Work out the finished part from the listing and answer in its coordinate system (mm). Round coordinates to 2 decimals unless told otherwise and drop trailing zeros. Loops run counter-clockwise (first coordinate to the right, second up) from the corner with the lowest first, then second, coordinate; pieces in that order, holes last. Notation, with made-up numbers: (58, -25.75) - (80, -25.75) arc R16 cw to (80, -19.75) - close; hole circle Ø10 at (74, 70). An arc over 180 degrees is marked (long way). Answer as CSV lines item,"result". Start each with the question number.
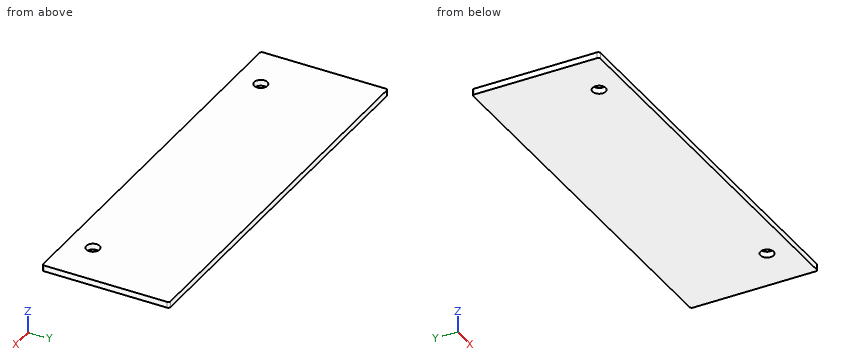
```python
from build123d import *

# Parameters (mm, degrees)
SKETCH_R  = 3.302
PAD_DEPTH = 3


with BuildPart() as part:
    # Sketch → Pad (new body)
    with BuildSketch(Plane.XY):
        with BuildLine():
            ThreePointArc((-98.21875, 31.75), (-98.925857, 31.457107), (-99.21875, 30.75))
            Line((-99.21875, -30.75), (-99.21875, 30.75))
            ThreePointArc((-99.21875, -30.75), (-98.925857, -31.457107), (-98.21875, -31.75))
            Line((98.21875, -31.75), (-98.21875, -31.75))
            ThreePointArc((98.21875, -31.75), (98.925857, -31.457107), (99.21875, -30.75))
            Line((99.21875, 30.75), (99.21875, -30.75))
            ThreePointArc((99.21875, 30.75), (98.925857, 31.457107), (98.21875, 31.75))
            Line((-98.21875, 31.75), (98.21875, 31.75))
        make_face()
        with Locations((-76.2, -19.05)):
            Circle(SKETCH_R, mode=Mode.SUBTRACT)
        with Locations((76.2, -19.05)):
            Circle(SKETCH_R, mode=Mode.SUBTRACT)
    extrude(amount=PAD_DEPTH)


solid = part.part
```
Item 1: Section B-B, the plane x = 76.2 is taken. Give the vertices of the cut face in (y, z), and give its area (3 significant figures).
Item 2: Section A-A, the plane y = -19.05 is taken. Give the vertices of the cut face in (x, z), and give its area (3 significant figures).
Item 3: Find the intervals of material crossed by L1, parallel to Y at x = 76.2, z = 1.65; L2, parallel to X at y = -17, z = 2.65, in increasing order.
Answer:
1,outline,"(-31.75, 0) - (-22.35, 0) - (-22.35, 3) - (-31.75, 3) - close; (-15.75, 0) - (31.75, 0) - (31.75, 3) - (-15.75, 3) - close"
1,area,"171 mm²"
2,outline,"(-99.22, 0) - (-79.5, 0) - (-79.5, 3) - (-99.22, 3) - close; (-72.9, 0) - (72.9, 0) - (72.9, 3) - (-72.9, 3) - close; (79.5, 0) - (99.22, 0) - (99.22, 3) - (79.5, 3) - close"
2,area,"556 mm²"
3,L1,"y = -31.75 to -22.35, -15.75 to 31.75"
3,L2,"x = -99.22 to -78.79, -73.61 to 73.61, 78.79 to 99.22"
